Check sheet for the drawn part. Datum: minimum x, y, z corner. Units: mm. A direction names the side the tool comes from. Coordinates: 2 decimals unless noted, no trailing zeros. Write each loop counter-clockwise with the first axis right and the second up, starting at its lowest first coordinate (ties: lowest second). Pieces come first, ordered by that corner, then holes. Notation, with made-up numbers: (12.5, -15.75) -> (41.5, -15.75) arc R20 ccw to (41.5, 20.25) -> close; hole circle Ø2 at (34.5, 17.25). An arc over 180 degrees is marked (long way). Answer in a Markdown table with one row per item. Add a question column.
Q1. Thickness scan on line 1 (X direction, y = 6.5, z = 14.25); line 2 (Z direction, x = 23.5, y = 32). Record the ranges inside material, lowest first.
Q2. Section check B-B, the plane z = 13.25. Record the boundary of the cut face in (x, y), and give its area (3 significant figures).
Q3. Section check C-C, the plane y = 4.5. Record the boundary of the cut face in (x, z), and give its area (3 significant figures).
Q4. Gauge pin test, flat ends, axial feed: P1, Ø1, axis at y = 36.5, z = 19.5, coming from the -X side; P2, Ø8, axis at y = 29, z = 7, coming from the +X side; P3, Ø10, axis at x = 40, z = 5, coming from the +Y side. Record the tip position at first contact, or that the pin passes through.
Q5. Tool access check on the marked faces 1, 2, 3, 4 and 5. Record the directions out of +Z, -Z, +X, -X, +Y, -Y that give a thin tool (end or side, any length) a straight path to the whole face; none if there is none.
Q6. Section check A-A, the plane x = 46. Record the boundary of the cut face in (y, z), and give its area (3 significant figures).
Q7. Release check for a two-part mould opening along Z. For the marked faces 6, 7, 8 and 9 record: pulls with the +Z half, pulls with the -Z half, needs draft (parallel to the pull), parting line crosses it, or undercut.
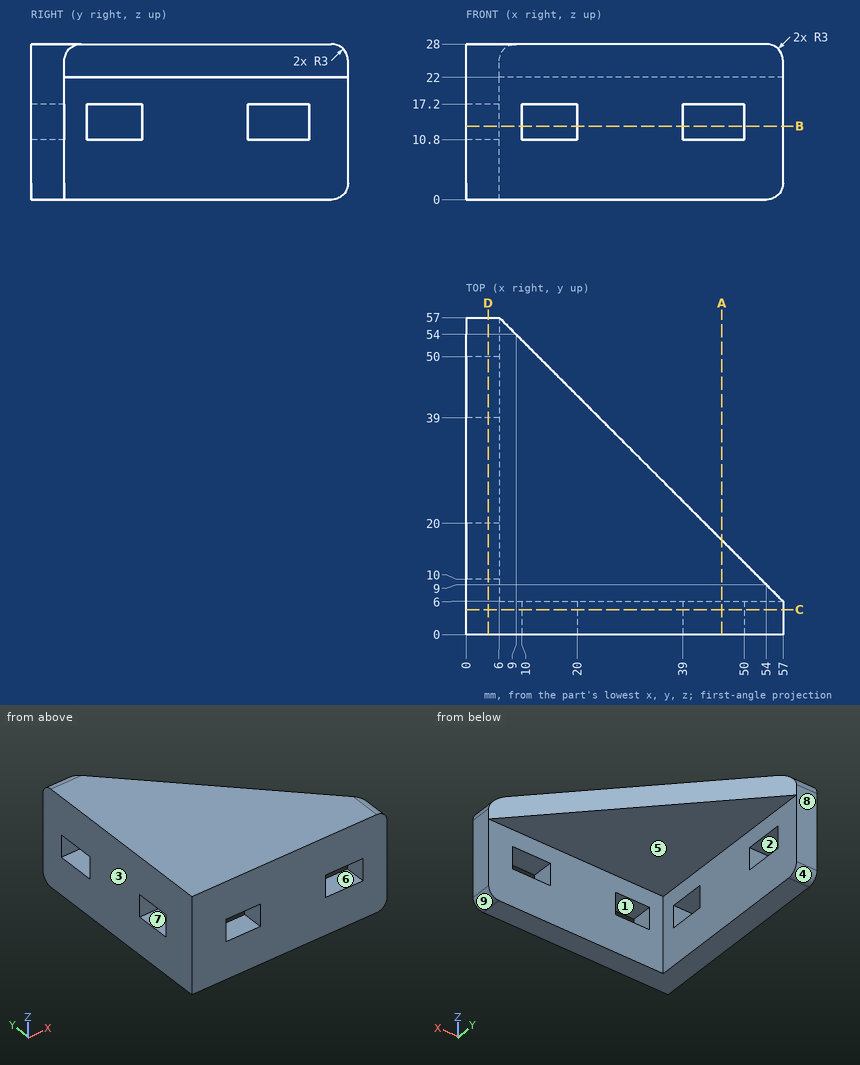
Calculated:
| question | item | result |
|---|---|---|
| 1 | line 1 | x = 0 to 6 |
| 1 | line 2 | z = 22 to 28 |
| 2 | outline | (0, 0) -> (10, 0) -> (10, 6) -> (6, 6) -> (6, 10) -> (0, 10) -> close; (0, 20) -> (6, 20) -> (6, 39) -> (0, 39) -> close; (0, 50) -> (6, 50) -> (6, 57) -> (0, 57) -> close; (20, 0) -> (39, 0) -> (39, 6) -> (20, 6) -> close; (50, 0) -> (57, 0) -> (57, 6) -> (50, 6) -> close |
| 2 | area | 396 mm² |
| 3 | outline | (0, 0) -> (54, 0) arc R3 ccw to (57, 3) -> (57, 25) arc R3 ccw to (54, 28) -> (0, 28) -> close; hole (10, 10.8) -> (20, 10.8) -> (20, 17.2) -> (10, 17.2) -> close; hole (39, 10.8) -> (50, 10.8) -> (50, 17.2) -> (39, 17.2) -> close |
| 3 | area | 1,460 mm² |
| 4 | P1 | stops at x = 0 |
| 4 | P2 | stops at x = 6 |
| 4 | P3 | stops at y = 6 |
| 5 | face 1 | +Y, -Y |
| 5 | face 2 | +X, -X |
| 5 | face 3 | +Z, -Z, -X, +Y, -Y |
| 5 | face 4 | -Z, +X, -X, +Y |
| 5 | face 5 | -Z, +X, +Y |
| 6 | outline | (0, 0) -> (6, 0) -> (6, 10.8) -> (0, 10.8) -> close; (0, 17.2) -> (6, 17.2) -> (6, 22) -> (17, 22) -> (17, 28) -> (0, 28) -> close |
| 6 | area | 196 mm² |
| 7 | face 6 | undercut |
| 7 | face 7 | undercut |
| 7 | face 8 | needs draft |
| 7 | face 9 | pulls with the -Z half |
